CAD build for the part. Positions are in the model's coordinates, mm. Round coordinates to 2 decimals unless told otherwise and drop trailing zeros.
```python
from build123d import *

# Parameters (mm, degrees)
BLANKSKE_W              = 110
BLANKSKE_H              = 11
BLANK_DEPTH             = 10
TOOTHCUTSIM_DEPTH       = 112
TEETHCUTS_COUNT         = 36
TEETHCUTS_PITCH         = 3.14159265
CUT_EXTRUDE1_DEPTH      = 112
CUT_EXTRUDE1_DEPTH_BACK = 112
SKETCH1_R               = 8.35
SKETCH3_W               = 2.609723718
SKETCH3_H               = 4.369414265
CUT_EXTRUDE2_DEPTH      = 10


with BuildPart() as part:
    # BlankSke → Blank (new body)
    with BuildSketch(Plane.XY):
        with Locations((55, 5.5)):
            Rectangle(BLANKSKE_W, BLANKSKE_H)
    extrude(amount=-BLANK_DEPTH)

    # TooCutSkeSim → ToothCutSim (cut, through all)
    with BuildSketch(Plane.XY):
        Polygon((0.576126182, 8.75), (-0.576126182, 8.75), (-1.164584633, 11.0254), (1.164584633, 11.0254), align=None)
    toothcutsim = extrude(amount=-TOOTHCUTSIM_DEPTH, mode=Mode.SUBTRACT)

    # TeethCuts: ToothCutSim ×36
    with Locations(*[(i * TEETHCUTS_PITCH, 0, 0) for i in range(1, TEETHCUTS_COUNT)]):
        add(toothcutsim, mode=Mode.SUBTRACT)

    # Sketch1 → Cut-Extrude1 (cut, two sides: drawn at the far end of the back side and taken through both)
    with BuildSketch(Plane(origin=(110, 0, 0), x_dir=(0, 0, -1), z_dir=(1, 0, 0)).offset(-CUT_EXTRUDE1_DEPTH_BACK)):
        with Locations((5, 0)):
            Circle(SKETCH1_R)
    extrude(amount=CUT_EXTRUDE1_DEPTH + CUT_EXTRUDE1_DEPTH_BACK, mode=Mode.SUBTRACT)

    # Sketch3 → Cut-Extrude2 (cut)
    with BuildSketch(Plane(origin=(0, 0, -10), x_dir=(-1, 0, 0), z_dir=(0, 0, -1))):
        with Locations((-108.695138141, 8.872195451)):
            Rectangle(SKETCH3_W, SKETCH3_H)
        Polygon((-0.576126182, 8.75), (-0.576126182, 11), (0, 11), (0, 6.687488318), (-0.576126182, 6.687488318), align=None)
    extrude(amount=-CUT_EXTRUDE2_DEPTH, mode=Mode.SUBTRACT)


solid = part.part
```
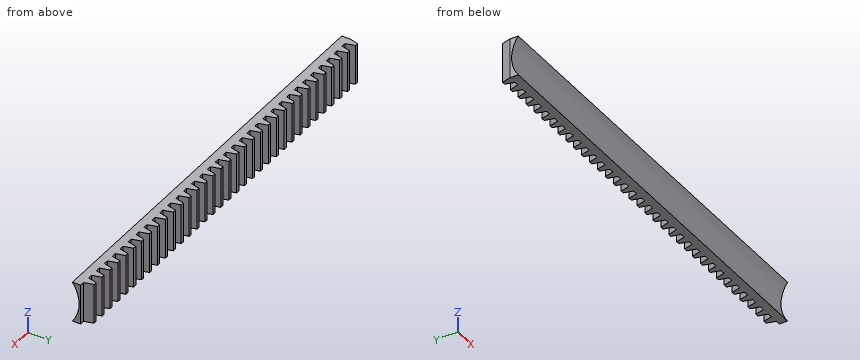
Item 1: Flat gauge pins, fed straight in: P1, Ø1, axis at x = 88, z = -8.5, coming from the -Y side; P2, Ø0.6, axis at x = 72.5, z = -5.5, coming from the +Y side; P3, Ø1, axis at y = 9.5, z = -7.5, coming from the -X side. Where does each tip first touch, or does it go through?
Answers follow:
P1: stops at y = 7.33
P2: stops at y = 8.75
P3: stops at x = 0.64
Item 2: Probe line 1 (Z direction, x = 9, y = 6.95); line 2 (Z direction, x = 67, y = 6.9); line 3 (Y direction, x = 22.5, z = -9.5). List the from-to ranges inside material, lowest first.
Answers follow:
line 1: z = -10 to -9.63, -0.37 to 0
line 2: z = -10 to -9.7, -0.3 to 0
line 3: y = 7.03 to 8.75
Item 3: Cut at A-A, the plane y = 9.4. State how many separate pieces and enclosed holes the cut face has, plus the area to 3 significant figures.
Answers follow:
separate pieces: 34
enclosed holes: 0
area: 562 mm2
